The listing builds one solid part. Answer for the finished solid, in the listing's coordinates (mm). A direction names the side the tool comes from. Round coordinates to 2 decimals unless told otherwise and drop trailing zeros. Loops run counter-clockwise (first coordinate to the right, second up) from the corner with the lowest first, then second, coordinate; pieces in that order, holes last. Notation, with made-up numbers: (-13, 57.5) - (30, 57.5) arc R27 ccw to (30, 91.5) - close; hole circle Ø6 at (-37.75, -24). An arc over 180 degrees is marked (long way). Write item = value, one per line. Start each with the question number.
1) A tool of negligible diameter and unlimited length cuts with its end or side. For faces 1 (the flat face through (145, 18, 26)), 2 (the flat face through (0, 1, 1)), from which of +Z, -Z, +X, -X, +Y, -Y can it reach the whole face along a straight path? Write none if from no direction.
2) Straight lines are drawn through the part: line 1 along Y through (x, z) = (175.8, -27); line 2 along X through (y, z) = (-2.5, 13); line 3 along X through (y, z) = (-34.5, -5). For each, find the intervals that lie inside material, in ascending order.
3) Section D-D, the plane x = 25 is taken. Determine the outline of the cut face in (y, z).
4) Given pin 1 Ø12 at (x, y) = (96, 32.5) entering from +Z; pin 2 Ø3 at (x, y) = (18, -8) entering from -Z; pin 3 Ø1.5 at (y, z) = (0, 35) entering from +X, each flat-ended and moving along its own axis, determine where each tip first touches the part or whether it passes through.
5) Section B-B, the plane x = 153 is taken. Determine the outline of the cut face in (y, z).
6) Section C-C, the plane z = 25.5 is taken. Determine the outline of the cut face in (x, y), and give its area (3 significant figures).
7) Section A-A, the plane z = 0 is taken. Determine the outline of the cut face in (x, y), and give its area (3 significant figures).
Autodesk Fusion 360 part; units mm, degrees
sketch "Sketch1" plane through (0, 0, 0) normal (1, 0, 0) x (0, 0, -1)
  line L0 (0, 0) -> (0, 45)
  line L1 (0, 0) -> (0, -45)
  line L2 (0, 45) -> (37.5, 45)
  line L3 (0, 45) -> (-37.5, 45)
  line L4 (0, -45) -> (37.5, -45)
  line L5 (0, -45) -> (-37.5, -45)
  arc A0 (-37.5, 45) -> (-37.5, -45) centre (79.119, 0) ccw
  arc A1 (37.5, -45) -> (37.5, 45) centre (-79.119, 0) ccw
  dimension "d1" = 45
  dimension "d2" = 45
  dimension "d3" = 37.5
  dimension "d4" = 37.5
  dimension "d5" = 37.5
  dimension "d6" = 37.5
  dimension "d8" = 125
extrude "Extrude1" add sketch "Sketch1" along normal blind 100
extrude "Extrude2" add 1 faces at (100, -15.2642, -14.2806) along direction (1, 0, 0) blind 35 draft -15
sketch "Sketch2" plane through (135, 0, 0) normal (1, 0, 0) x (0, 0, -1)
  line L0 (-30.8786, -35.6218) -> (30.8786, -35.6218)
  arc A0 (30.8786, -35.6218) -> (30.8786, 35.6218) centre (-79.119, 0) ccw
  line L1 (30.8786, 35.6218) -> (-30.8786, 35.6218)
  arc A1 (-30.8786, 35.6218) -> (-30.8786, -35.6218) centre (79.119, 0) ccw
  circle A2 centre (0, 0) radius 34.5
  dimension "d13" = 69
extrude "Extrude3" add sketch "Sketch2" along normal blind 10 contours A2
sketch "Sketch3" plane through (145, 0, 0) normal (1, 0, 0) x (0, 0, -1)
  circle A0 centre (0, 0) radius 34.5
  circle A1 centre (0, 0) radius 31
  dimension "d16" = 62
extrude "Extrude4" add sketch "Sketch3" along normal blind 30 contours A1
sketch "Sketch4" plane through (175, 0, 0) normal (1, 0, 0) x (0, 0, -1)
  circle A0 centre (0, 0) radius 31
  line L0 (0, 0) -> (27, 0)
  circle A1 centre (27, 0) radius 2.5
  circle A2 centre (27, 0) radius 1.5
  dimension "d19" = 27
  dimension "d20" = 5
  dimension "d21" = -1
extrude "Extrude5" add sketch "Sketch4" along normal blind 1 contours A1
Geometry check:
q1.face_1 = +X
q1.face_2 = +Z, -Z, -X, +Y, -Y
q2.line_1 = -2.5 to -1.5, 1.5 to 2.5
q2.line_2 = 0 to 175
q2.line_3 = 0 to 135
q3.outline = (-45, -37.5) arc R125 ccw to (45, -37.5) - (45, 37.5) arc R125 ccw to (-45, 37.5) - close
q4.pin_1 = 43.04
q4.pin_2 = -45.71
q4.pin_3 = 145
q5.outline = circle Ø62 at (0, 0)
q6.outline = (0, -45) - (100, -45) - (135, -35.62) - (135, -23.24) - (145, -23.24) - (145, -17.63) - (175, -17.63) - (175, 17.63) - (145, 17.63) - (145, 23.24) - (135, 23.24) - (135, 35.62) - (100, 45) - (0, 45) - close
q6.area = 13,300 mm2
q7.outline = (0, -45) - (100, -45) - (135, -35.62) - (135, -34.5) - (145, -34.5) - (145, -31) - (175, -31) - (175, 31) - (145, 31) - (145, 34.5) - (135, 34.5) - (135, 35.62) - (100, 45) - (0, 45) - close
q7.area = 14,400 mm2
